from build123d import *

# Parameters (mm, degrees)
SKETCH1_W                      = 100
SKETCH1_H                      = 55
BOSS_EXTRUDE1_DEPTH            = 25
CUT_EXTRUDE1_DEPTH             = 26
CUT_EXTRUDE2_DEPTH             = 101
CUT_EXTRUDE3_DEPTH             = 56
M5X0_8_TAPPED_HOLE1_AT_2_COUNT = 2
M5X0_8_TAPPED_HOLE1_AT_2_PITCH = 19.5
M5X0_8_TAPPED_HOLE1_AT_3_COUNT = 2
M5X0_8_TAPPED_HOLE1_AT_3_PITCH = 39


with BuildPart() as part:
    # Sketch1 → Boss-Extrude1 (new body)
    with BuildSketch(Plane(origin=(0, 0, 0), x_dir=(1, 0, 0), z_dir=(0, 1, 0))):
        Rectangle(SKETCH1_W, SKETCH1_H)
    extrude(amount=BOSS_EXTRUDE1_DEPTH)

    # Sketch2 → Cut-Extrude1 (cut, through all)
    with BuildSketch(Plane(origin=(0, 25, 0), x_dir=(1, 0, 0), z_dir=(0, 1, 0))):
        with BuildLine():
            Line((-35, -14), (35, -14))
            ThreePointArc((35, -14), (38.535533906, -12.535533906), (40, -9))
            Line((40, -9), (40, 9))
            ThreePointArc((40, 9), (38.535533906, 12.535533906), (35, 14))
            Line((35, 14), (-35, 14))
            ThreePointArc((-35, 14), (-38.535533906, 12.535533906), (-40, 9))
            Line((-40, 9), (-40, -9))
            ThreePointArc((-40, -9), (-38.535533906, -12.535533906), (-35, -14))
        make_face()
    extrude(amount=-CUT_EXTRUDE1_DEPTH, mode=Mode.SUBTRACT)

    # Sketch3 → Cut-Extrude2 (cut, through all)
    with BuildSketch(Plane(origin=(50, 0, 0), x_dir=(0, 0, -1), z_dir=(1, 0, 0))):
        Polygon((15.5, 25), (18.5, 19), (-18.5, 19), (-15.5, 25), align=None)
    extrude(amount=-CUT_EXTRUDE2_DEPTH, mode=Mode.SUBTRACT)

    # Sketch4 → Cut-Extrude3 (cut, through all)
    with BuildSketch(Plane.XY.offset(27.5)):
        with BuildLine():
            Line((-29, 14.5), (29, 14.5))
            ThreePointArc((29, 14.5), (34, 9.5), (29, 4.5))
            Line((29, 4.5), (-29, 4.5))
            ThreePointArc((-29, 4.5), (-34, 9.5), (-29, 14.5))
        make_face()
    extrude(amount=-CUT_EXTRUDE3_DEPTH, mode=Mode.SUBTRACT)

    # Sketch7 → M5x0.8 Tapped Hole1 (revolve, cut)
    with BuildSketch(Plane(origin=(50, 6, 19.5), x_dir=(0, 0, -1), z_dir=(0, 1, 0))):
        Polygon((0, 0), (0, 8.7618073), (2.1, 7.5), (2.1, 0), align=None)
    m5x0_8_tapped_hole1 = revolve(axis=Axis((56.35, 6, 19.5), (-1, 0, 0)), mode=Mode.SUBTRACT)

    # M5x0.8 Tapped Hole1 at 2: M5x0.8 Tapped Hole1 ×2
    with Locations(*[(0, 0, -i * M5X0_8_TAPPED_HOLE1_AT_2_PITCH) for i in range(1, M5X0_8_TAPPED_HOLE1_AT_2_COUNT)]):
        add(m5x0_8_tapped_hole1, mode=Mode.SUBTRACT)

    # M5x0.8 Tapped Hole1 at 3: M5x0.8 Tapped Hole1 ×2
    with Locations(*[(0, 0, -i * M5X0_8_TAPPED_HOLE1_AT_3_PITCH) for i in range(1, M5X0_8_TAPPED_HOLE1_AT_3_COUNT)]):
        add(m5x0_8_tapped_hole1, mode=Mode.SUBTRACT)

    # Mirror1: M5x0.8 Tapped Hole1 across plane
    add(m5x0_8_tapped_hole1.mirror(Plane(origin=(0, 0, 0), x_dir=(0, 0, 1), z_dir=(1, 0, 0))), mode=Mode.SUBTRACT)

    # Mirror1 copy 1 sketch → Mirror1 copy 1 (revolve, cut)
    with BuildSketch(Plane(origin=(-50, 6, 0), x_dir=(0, 0, -1), z_dir=(0, 1, 0))):
        Polygon((0, 0), (0, -8.7618073), (2.1, -7.5), (2.1, 0), align=None)
    revolve(axis=Axis((-56.35, 6, 0), (-1, 0, 0)), mode=Mode.SUBTRACT)

    # Mirror1 copy 2 sketch → Mirror1 copy 2 (revolve, cut)
    with BuildSketch(Plane(origin=(-50, 6, -19.5), x_dir=(0, 0, -1), z_dir=(0, 1, 0))):
        Polygon((0, 0), (0, -8.7618073), (2.1, -7.5), (2.1, 0), align=None)
    revolve(axis=Axis((-56.35, 6, -19.5), (-1, 0, 0)), mode=Mode.SUBTRACT)


solid = part.part
Verification items for the finished model (mm, model axes). A direction names the side the tool comes from. Give positions to 0.01 mm unless a question says otherwise; leave off trailing zeros. Order: outer loops, then holes, each group sorted by start corner. A loop starts at its lowest first (then second) coordinate and runs counter-clockwise, first axis right, second up. Notation, with made-up numbers: M 61.25,-7.75 L 114.25,-7.75 A5 cw 114.25,-1.75 Z; hole C 51,-5 d7. An arc over 180 degrees is marked long. Use one line per item in the form item = value. Start each with the question number.
Q1. Section check A-A (y = 9.5). Enter the section's corners in (x, z), then the cut area to 3 significant figures.
Q2. Scan lines: line 1 along Z through (x, y) = (48.75, 6); line 2 along Y through (x, z) = (26, 25); line 3 along Y through (x, z) = (46.5, 0). Record each from-to range of solid material in increasing order. Write a range as [from, to].
Q3. Go/stop test with flat-tipped pins: pin 1 Ø2.5 at (y, z) = (6, 0) entering from -X; pin 2 Ø3.5 at (y, z) = (6, -19.5) entering from +X; pin 3 Ø4 at (y, z) = (6, 19.5) entering from +X. Record where each tip stops, or that it passes through.
Q4. Access from +Z, -Z, +X, -X, +Y, -Y to the whole of each face (thin tool, end or side, straight path). Record for faces 1 (the cylindrical face through (38, 10, 13)), 2 (the flat face through (1, 22, -17)), 3 (the cylindrical face through (-34, 9.4, -20.7)), 4 (the cylindrical face through (46.302, 7.863, -0.969)).
Q5. Section check B-B (x = -3). Enter the section's corners in (y, z).
Q6. Mould release check, pull along Z, two halves, no side actions. Record for faces 5 (the flat face through (0, 16, -14)), 6 (the flat face through (-1, 25, -22)), 7 (the conical face through (41.46, 5.75, 19.77)): +Z half, -Z half, draft (parallel to the pull), parting line (faces both ways), or undercut.
Q7. Section check C-C (y = 23). Enter the section's corners in (x, z), then the cut area to 3 significant figures.
Evaluation:
q1.outline = M -50,-27.5 L -34,-27.5 L -34,-14 L -35,-14 A5 cw -40,-9 L -40,9 A5 cw -35,14 L -34,14 L -34,27.5 L -50,27.5 Z; M 34,-27.5 L 50,-27.5 L 50,27.5 L 34,27.5 L 34,14 L 35,14 A5 cw 40,9 L 40,-9 A5 cw 35,-14 L 34,-14 Z
q1.area = 1,450 mm2
q2.line_1 = [-27.5, -21.6], [-17.4, -2.1], [2.1, 17.4], [21.6, 27.5]
q2.line_2 = [0, 4.5], [14.5, 25]
q2.line_3 = [0, 3.9], [8.1, 19]
q3.pin_1 = -41.99
q3.pin_2 = 42.29
q3.pin_3 = 42.44
q4.face_1 = +Y, -Y
q4.face_2 = +X, -X
q4.face_3 = +Z, -Z
q4.face_4 = +X
q5.outline = M 0,-27.5 L 4.5,-27.5 L 4.5,-14 L 0,-14 Z; M 0,14 L 4.5,14 L 4.5,27.5 L 0,27.5 Z; M 14.5,-27.5 L 25,-27.5 L 25,-15.5 L 19,-18.5 L 19,-14 L 14.5,-14 Z; M 14.5,14 L 19,14 L 19,18.5 L 25,15.5 L 25,27.5 L 14.5,27.5 Z
q6.face_5 = undercut
q6.face_6 = draft
q6.face_7 = undercut
q7.outline = M -50,-27.5 L 50,-27.5 L 50,-16.5 L -50,-16.5 Z; M -50,16.5 L 50,16.5 L 50,27.5 L -50,27.5 Z
q7.area = 2,200 mm2
